Design review of the part built by this model. Coordinates are the model's own, in mm. A direction names the side the tool comes from. Give positions to 0.01 mm unless a question says otherwise; leave off trailing zeros. Order: outer loops, then holes, each group sorted by start corner. A loop starts at its lowest first (then second) coordinate and runs counter-clockwise, first axis right, second up. Notation, with made-up numbers: (-7, -21) -> (30, -21) arc R20 cw to (30, -8) -> close; hole circle Ø11 at (5.5, 28.5). An arc over 180 degrees is marked (long way). Return JSON: item names as keys, results as strings.
Autodesk Fusion 360 part; units mm, degrees
sketch "Sketch1" plane through (0, 0, 0) normal (0, 1, 0) x (1, 0, 0)
  line L0 (32.5, 9.65) -> (-32.5, 9.65)
  line L1 (-32.5, 9.65) -> (-32.5, -9.65)
  line L2 (-32.5, -9.65) -> (32.5, -9.65)
  line L3 (32.5, -9.65) -> (32.5, 9.65)
  line L4 (32.5, 9.65) -> (-32.5, -9.65) construction
  line L5 (-32.5, 9.65) -> (32.5, -9.65) construction
  line L6 (32.5, 9.65) -> (34.5, 9.65)
  line L7 (34.5, 9.65) -> (34.5, -9.35)
  line L8 (34.5, -9.35) -> (32.5, -9.35)
  line L9 (32.5, -9.35) -> (32.5, 9.65)
  line L10 (-32.5, 9.65) -> (-37.5, 9.65)
  line L11 (-37.5, 9.65) -> (-37.5, -9.5)
  line L12 (-37.5, -9.5) -> (-32.5, -9.5)
  line L13 (-32.5, -9.5) -> (-32.5, 9.65)
  dimension "d1" = 65
  dimension "d2" = 19.3
  dimension "d3" = 2
  dimension "d4" = 19
  dimension "d5" = 5
extrude "Extrude1" add sketch "Sketch1" along normal blind 5.5 contours L0 L1 L2 L3 L9 L13
extrude "Extrude2" add sketch "Sketch1" along normal blind 2 contours L3 L6 L7 L8 L9
extrude "Extrude3" add sketch "Sketch1" along normal blind 2 contours L1 L10 L11 L12 L13
sketch "Sketch2" plane through (0, 0, 9.65) normal (0, 0, 1) x (1, 0, 0)
  line L0 (-32.5, 0) -> (32.5, 0)
  line L1 (34.5, 0) -> (34.5, 2)
  line L2 (34.5, 2) -> (32.5, 2)
  line L3 (32.5, 0) -> (32.5, 5.5)
  line L4 (32.5, 5.5) -> (-32.5, 5.5)
  line L5 (-32.5, 5.5) -> (-32.5, 0)
  line L6 (-32.5, 2) -> (-37.5, 2)
  line L7 (-37.5, 2) -> (-37.5, 0)
  line L8 (33.6424, 5.5) -> (42.1424, 5.5)
  line L9 (33.6424, 5.5) -> (33.6424, 2.4499)
  line L10 (42.1424, 5.5) -> (42.1424, 2.4499)
  line L11 (42.1424, 2.4499) -> (33.6424, 2.4499)
  line L12 (-32.5, 0) -> (-40.5, 0)
  line L13 (-45.0976, 3.4495) -> (-41.0979, 3.4562)
  line L14 (-40.5987, 3.957) -> (-40.6027, 6.3116)
  line L15 (-42.5164, 5.4956) -> (-45.1003, 5.4913)
  line L16 (-45.5995, 4.9908) -> (-45.5984, 3.949)
  line L17 (-37.5, 2) -> (-39.8153, 7.5767)
  line L18 (-40.1899, 7.5627) -> (-40.6027, 6.3116)
  arc A0 (-39.8153, 7.5767) -> (-40.1899, 7.5627) centre (-40, 7.5) ccw
  arc A1 (-45.1003, 5.4913) -> (-45.5995, 4.9908) centre (-45.0995, 4.9913) ccw
  arc A2 (-45.5984, 3.949) -> (-45.0976, 3.4495) centre (-45.0984, 3.9495) ccw
  arc A3 (-41.0979, 3.4562) -> (-40.5987, 3.957) centre (-41.0987, 3.9562) ccw
  line L19 (33.6424, 2.4499) -> (33.6424, 2)
  line L20 (-35.4489, 2) -> (-36.9951, 9.0494)
  arc A4 (-36.9951, 9.0494) -> (-42.0393, 8.86) centre (-39.5001, 8.4999) ccw
  line L21 (-42.0393, 8.86) -> (-42.5164, 5.4956)
  line L22 (32.5, 0) -> (34.5, 0)
  line L23 (32.5, 2) -> (32.5, 0)
  line L24 (-37.5, 0) -> (-32.5, 0)
  line L25 (-32.5, 0) -> (-32.5, 2)
  line L26 (34.5, 2) -> (34.5, 2.4499)
  point P0 (-45.5979, 3.4487)
  point P1 (-40.5979, 3.457)
  dimension "d12" = 8.5
  dimension "d41" = 8
  dimension "d42" = 5
  dimension "d44" = 0.2
  dimension "d45" = 0.5
  dimension "d46" = 0.5
  dimension "d47" = 0.5
extrude "Extrude4" add sketch "Sketch2" against normal blind 19.2 contours L1 L2 L3 L22 L23 | L2 L11 L19 L26 | L8 L9 L10 L11
extrude "Extrude5" add sketch "Sketch2" along normal blind -19.3 and the other way blind 2.5 contours L5 L6 L7 L12 L24 L25 | L1 L2 L3 L22 L23 | L2 L11 L19 L26 | L8 L9 L10 L11
fillet "Fillet1" radius 1 1 edges at (-32.5, 5.5, 0)
fillet "Fillet2" radius 1 1 edges at (32.5, 5.5, 0)
sketch "Sketch3" plane through (0, 5.5, 0) normal (0, 1, 0) x (-1, 0, 0)
  line L0 (-33.6424, 9.65) -> (-42.1424, 9.65)
  line L1 (-42.1424, 9.65) -> (-42.1424, -9.65)
  line L2 (-42.1424, -9.65) -> (-33.6424, -9.65)
  line L3 (-33.6424, -9.65) -> (-33.6424, 9.65)
  line L4 (-33.6424, 0) -> (-42.1424, 0)
  circle A0 centre (-37.8924, -4.75) radius 1.5
  circle A1 centre (-37.8924, -4.75) radius 2.5
  circle A2 centre (-37.8924, 4.75) radius 2.5
  circle A3 centre (-37.8924, 4.75) radius 1.5
  dimension "d31" = 3
  dimension "d32" = 5
extrude "Extrude6" cut sketch "Sketch3" against normal blind 6 contours A0 | A3
extrude "Extrude10" add 1 faces at (34.5, 1.4833, 3.2167) along direction (1, 0, 0) blind 7.642
extrude "Extrude7" cut sketch "Sketch3" along normal blind -5.5 and the other way blind 1.5 contours A0 | A1 | A2 | A3
sketch "Sketch6" plane through (0, 5.5, 0) normal (0, 1, 0) x (-1, 0, 0)
  line L0 (-31.5, 9.65) -> (-31.5, -9.65)
  line L1 (-31.5, -9.65) -> (31.5, -9.65)
  line L2 (31.5, -9.65) -> (31.5, 9.65)
  line L3 (31.5, 9.65) -> (-31.5, 9.65)
  line L4 (31.5, 9.65) -> (-31.5, 9.65)
  line L5 (-31.5, 9.65) -> (-31.5, -9.65)
  line L6 (-31.5, -9.65) -> (31.5, -9.65)
  line L7 (31.5, -9.65) -> (31.5, 9.65)
  line L8 (-29, -7.15) -> (29, -7.15)
  line L9 (29, -9.65) -> (29, 9.65)
  line L10 (29, 7.15) -> (-29, 7.15)
  line L11 (-29, 7.15) -> (-29, -7.15)
  line L12 (-26.5, 7.15) -> (-26.5, -7.15)
  line L13 (-29, 7.15) -> (-29, 9.65)
  line L14 (-29, -7.15) -> (-29, -9.65)
  line L15 (-31.5, 9.65) -> (-32.5, 9.65)
  line L16 (-32.5, 9.65) -> (-32.5, -9.65)
  line L17 (-32.5, -9.65) -> (-31.5, -9.65)
  line L18 (31.5, -9.65) -> (32.5, -9.65)
  line L19 (32.5, -9.65) -> (32.5, 9.65)
  line L20 (32.5, 9.65) -> (31.5, 9.65)
  line L21 (31.5, 9.65) -> (31.5, -9.65)
  line L22 (26.5, -7.15) -> (26.5, 7.15)
  line L23 (29, 0) -> (29, 7.15)
  dimension "d58" = -2.5
  dimension "d69" = -2.5
extrude "Extrude11" cut sketch "Sketch6" against normal blind 2.5 contours L8 L10 L12 L22
extrude "Extrude12" cut sketch "Sketch6" against normal blind 3.5 contours L0 L1 L3 L4 L5 L6 L11 L13 L14 | L0 L5 L15 L16 L17 | L1 L2 L3 L4 L6 L7 L9 L21 L23 | L2 L7 L18 L19 L20 L21
fillet "Fillet4" radius 1 1 edges at (29, 5.5, 0)
extrude "Extrude14" add sketch "Sketch2" along normal blind -16.55 and the other way blind 2.75 contours L5 L6 L7 L12 L24 L25 | L6 L13 L14 L15 L16 L17 L18 A0 A1 A2 A3 L20 A4 L21
extrude "Extrude15" add sketch "Sketch2" against normal blind 0.8 contours L5 L6 L7 L12 L24 L25
fillet "Fillet5" radius 2 2 edges at (33.6424, 2, 0) (29, 2, 0)
fillet "Fillet6" radius 2 2 edges at (-35.4489, 2, 0) (-29, 2, 0)
extrude "Extrude16" add 1 faces at (-13.1932, 0, 1.4591) along direction (0, -1, 0) blind 0.4
sketch "Sketch8" plane through (0, 0, 6.9) normal (0, 0, 1) x (1, 0, 0)
  line L0 (-37.5, 2) -> (-33.84, 2)
  arc A0 (-35.7936, 3.5715) -> (-33.84, 2) centre (-33.84, 4) ccw
  line L1 (-35.7936, 3.5715) -> (-36.9951, 9.0494)
  arc A1 (-36.9951, 9.0494) -> (-42.0393, 8.86) centre (-39.5001, 8.4999) ccw
  line L2 (-42.0393, 8.86) -> (-42.5164, 5.4956)
  line L3 (-42.5164, 5.4956) -> (-45.1003, 5.4913)
  arc A2 (-45.1003, 5.4913) -> (-45.5995, 4.9908) centre (-45.0995, 4.9913) ccw
  line L4 (-45.5995, 4.9908) -> (-45.5984, 3.949)
  arc A3 (-45.5984, 3.949) -> (-45.0976, 3.4495) centre (-45.0984, 3.9495) ccw
  line L5 (-45.0976, 3.4495) -> (-41.0979, 3.4562)
  arc A4 (-41.0979, 3.4562) -> (-40.5987, 3.957) centre (-41.0987, 3.9562) ccw
  line L6 (-40.5987, 3.957) -> (-40.6027, 6.3116)
  line L7 (-40.6027, 6.3116) -> (-40.1899, 7.5627)
  arc A5 (-39.8153, 7.5767) -> (-40.1899, 7.5627) centre (-40, 7.5) ccw
  line L8 (-39.8153, 7.5767) -> (-37.5, 2)
  line L9 (-40, 6.5) -> (-46.4842, 6.4892)
  line L10 (-46.4842, 6.4892) -> (-46.4774, 2.362)
  line L11 (-46.4774, 2.362) -> (-39.9747, 2.3728)
  line L12 (-39.9747, 2.3728) -> (-40, 6.5)
extrude "Extrude17" cut sketch "Sketch8" against normal blind 2 contours L2 L3 A2 L4 A3 L5 A4 L6 L7 L9 L10 L11 L12 | L2 L3 A2 L4 A3 L5 A4 L6 L7 L9
extrude "Extrude18" cut sketch "Sketch8" along normal blind -13.8 and the other way blind 11.8 contours L2 L3 A2 L4 A3 L5 A4 L6 L7 L9 L10 L11 L12 | L2 L3 A2 L4 A3 L5 A4 L6 L7 L9
Item 1: Add section C-C (x = -35). Give the boundary of the cut face in (y, z), plus the area to 3 significant figures.
Result set:
{"outline": "(-0.4, -9.65) -> (2, -9.65) -> (2, -6.9) -> (2.37, -6.9) -> (2.37, 6.9) -> (2, 6.9) -> (2, 9.65) -> (-0.4, 9.65) -> close", "area": "51.4 mm^2"}
Item 2: Add section B-B (x = -11.5). Give the boundary of the cut face in (y, z).
Result set:
{"outline": "(-0.4, -9.65) -> (5.5, -9.65) -> (5.5, -7.15) -> (3, -7.15) -> (3, 7.15) -> (5.5, 7.15) -> (5.5, 9.65) -> (-0.4, 9.65) -> close"}
Item 3: Mouldability with a two-part tool opening along Z and no side actions: class faces 1 (the face through (26.5, 4, 0)), 2 (the face through (33.07, 2.6, -0.14)), 3 (the face through (-43, 5, -4.9)), 4 (the face through (2, 3, 9.65)) as released by +Z, released by -Z, zero draft, split by the parting line, or undercut.
Result set:
{"face 1": "undercut", "face 2": "zero draft", "face 3": "released by -Z", "face 4": "released by +Z"}
Item 4: For pin 1 (9.5 mm diameter, centred on x = 36, z = 3.5, fed in from +Y); pin 2 (2.5 mm diameter, centred on x = -37, y = 5.5, fed in from +Z); pin 3 (1.5 mm diameter, centred on x = 37.5, z = -3.5, fed in from -Y), all flat-tipped, find the tip position at first contact; note any pin that passes through.
Result set:
{"pin 1": "stops at y = 5.5", "pin 2": "stops at z = 6.9", "pin 3": "stops at y = 4"}
Item 5: Wall thickness on L1, parallel to Z at x = -19, y = 5.25; L2, parallel to X at y = 3.25, z = 6.5; L3, parallel to X at y = 4.25, z = 0: over which ranges is each line inside the solid? List them lowest first. Write a range as [from, to].
Result set:
{"L1": "z = [-9.65, -7.15], [7.15, 9.65]", "L2": "x = [-38.02, -35.69], [-29.15, -26.5], [26.5, 29.15], [33.5, 36.11], [39.68, 42.14]", "L3": "x = [-45.6, -40.6], [-38.43, -35.94], [-29, -26.5], [26.5, 29], [33.64, 42.14]"}
Item 6: Machinability: for faces 5 (the face through (-1, 5.5, -8)), 6 (the face through (38, 4, 3)), 7 (the face through (-43, 5, 4.9)), 8 (the face through (33.642, 5, 0)), which of the approach directions +Z, -Z, +X, -X, +Y, -Y give a long, thin tool a straight path to every point of the face, cutting with its end or side? Answer none if there is none.
Result set:
{"face 5": "+Z, -Z, +X, +Y", "face 6": "-Y", "face 7": "+Z, -X, -Y", "face 8": "+Z, -Z, +Y"}
